Check sheet for the modelled part. Datum: model origin and axes. Units: mm. A direction names the side the tool comes from. Round coordinates to 2 decimals unless told otherwise and drop trailing zeros. Write each loop counter-clockwise with the first axis right and the second up, starting at its lowest first coordinate (ties: lowest second). Pieces come first, ordered by that corner, then holes.
Item 1: Tool access check on faces 4 (the flat face through (165, 5, -10)), 5 (the flat face through (-165, 5, -10)), 6 (the cylindrical face through (-162.535, 10.382, -19.961)), 7 (the flat face through (-200, 0, 0)), 8 (the cylindrical face through (82.35, -2.17, -9.76)). Record the directions out of +Z, -Z, +X, -X, +Y, -Y that give a thin tool (end or side, any length) a straight path to the whole face; none if there is none.
Item 2: Cross-section at D-D on x = -155.5. Enter the section's corners in (y, z), plus the area to 3 significant figures.
Item 3: Cross-section at A-A on z = 17.5. Enter the section's corners in (x, y), plus the area to 3 significant figures.
Item 4: Cross-section at B-B on y = -14. Enter the section's corners in (x, z), plus the area to 3 significant figures.
Item 5: Cross-section at C-C on z = 0. Enter the section's corners in (x, y), plus the area to 4 significant figures.
Item 6: Go/stop test with flat-tipped pins: pin 1 Ø5 at (y, z) = (2, -18) entering from -X; pin 2 Ø3 at (x, y) = (-98, 4.5) entering from -Z; pin 3 Ø4 at (y, z) = (-10.5, 6) entering from +X. Record where each tip stops, or that it passes through.
Item 7: Material ranges on line 1 (X direction, y = 18, z = 13); line 2 (Y direction, x = -91, z = 1); line 3 (Z direction, x = 90, y = -0.5), recorded low to high.
Item 8: Release check for a two-part mould opening along X. For faces 1 (the cylindrical face through (0.035, 10.382, -19.961)), 2 (the flat face through (200, 0, 0)), 3 (the cylindrical face through (-80.15, -2.17, -9.76)) record: +X half, -X half, draft (parallel to the pull), parting line (faces both ways), or undercut.
from build123d import *

# Parameters (mm, degrees)
F0_R     = 10
F1_DEPTH = 200
F4_R     = 22.5
F5_DEPTH = 5
F6_R     = 22.5
F7_DEPTH = 5
F8_R     = 22.5
F9_DEPTH = 2.5


with BuildPart() as f1:
    # F0 (on Right) → F1 (new body, symmetric)
    with BuildSketch(Plane.YZ):
        Circle(F0_R)
    extrude(amount=F1_DEPTH, both=True)

    # F4 (on offset) → F5 (join)
    with BuildSketch(Plane.YZ.offset(165)):
        Circle(F4_R)
    extrude(amount=-F5_DEPTH)

    # F6 (on offset) → F7 (join)
    with BuildSketch(Plane.YZ.offset(-165)):
        Circle(F6_R)
    extrude(amount=F7_DEPTH)

    # F8 (on Right) → F9 (join, symmetric)
    with BuildSketch(Plane.YZ):
        Circle(F8_R)
    extrude(amount=F9_DEPTH, both=True)


solid = f1.part
Response values:
1. face 4: +X
1. face 5: -X
1. face 6: +X, -X
1. face 7: +Z, -Z, -X, +Y, -Y
1. face 8: none
2. outline: circle Ø20 at (0, 0)
2. area: 314 mm2
3. outline: (-165, -14.14) - (-160, -14.14) - (-160, 14.14) - (-165, 14.14) - close; (-2.5, -14.14) - (2.5, -14.14) - (2.5, 14.14) - (-2.5, 14.14) - close; (160, -14.14) - (165, -14.14) - (165, 14.14) - (160, 14.14) - close
3. area: 424 mm2
4. outline: (-165, -17.61) - (-160, -17.61) - (-160, 17.61) - (-165, 17.61) - close; (-2.5, -17.61) - (2.5, -17.61) - (2.5, 17.61) - (-2.5, 17.61) - close; (160, -17.61) - (165, -17.61) - (165, 17.61) - (160, 17.61) - close
4. area: 528 mm2
5. outline: (-200, -10) - (-165, -10) - (-165, -22.5) - (-160, -22.5) - (-160, -10) - (-2.5, -10) - (-2.5, -22.5) - (2.5, -22.5) - (2.5, -10) - (160, -10) - (160, -22.5) - (165, -22.5) - (165, -10) - (200, -10) - (200, 10) - (165, 10) - (165, 22.5) - (160, 22.5) - (160, 10) - (2.5, 10) - (2.5, 22.5) - (-2.5, 22.5) - (-2.5, 10) - (-160, 10) - (-160, 22.5) - (-165, 22.5) - (-165, 10) - (-200, 10) - close
5. area: 8,375 mm2
6. pin 1: stops at x = -165
6. pin 2: stops at z = -9.54
6. pin 3: stops at x = 165
7. line 1: x = -165 to -160, -2.5 to 2.5, 160 to 165
7. line 2: y = -9.95 to 9.95
7. line 3: z = -9.99 to 9.99
8. face 1: draft
8. face 2: +X half
8. face 3: undercut
